Can you work these out from the model? Positions are in its coordinate system, mm. A direction names the side the tool comes from. Give positions to 0.01 mm unless a question says otherwise; leave off trailing zeros. Write each loop counter-clockwise with the first axis right and the second up, starting at its lowest first coordinate (ties: lowest second). Pieces come first, ordered by that corner, then holes.
1. Suppose I cut it at B-B (x = 1.75). Please give me the cut outline in (y, z), and give its area (3 significant figures).
2. Thinking about a two-plate mould opening in Z: for faces 3 (the flat face through (2, -4, 115.167)), 4 (the flat face through (2, -43.98, 30)), 5 (the cylindrical face through (1.6, 5.9, 103.3)), 6 (the cylindrical face through (1.6, 5.9, 27.1)), which applies, pulls with the +Z half, pulls with the -Z half, needs draft (parallel to the pull), parting line crosses it, or undercut?
3. I'm going to push a flat-ended pin straight in: pin 1 (3 mm diameter, centred on y = -31.21, z = 54.84, fed in from +X). Where does the tip first touch, or does it pass through?
4. Suppose I cut it at A-A (z = -11). Please give me the cut outline in (x, y) (3 decimals), and give its area (3 significant figures).
5. On a 3-axis mill with a long thin cutter (end or side, diameter ignored), from which of +Z, -Z, +X, -X, +Y, -Y can I reach the whole of each face in a straight line? I mean faces 1 (the flat face through (2, 44.989, 31)), 2 (the flat face through (2, -24.93, 30)). Say none if no direction works.
6. If I drill on probe 1 along Y at (x, z) = (1.15, -33); probe 2 along Z at (x, y) = (3.05, 8); probe 3 along Z at (x, y) = (2, 41.5), over which ranges is the centre line in solid material (lowest first)?
```python
from build123d import *

# Parameters (mm, degrees)
SKETCH1_R           = 2.54
BOSS_EXTRUDE1_DEPTH = 3.175


with BuildPart() as part:
    # Sketch1 → Boss-Extrude1 (new body)
    with BuildSketch(Plane(origin=(0, 0, 0), x_dir=(0, 0, -1), z_dir=(1, 0, 0))):
        Polygon((53.108364313, 44.988743573), (-118.341635687, 44.988743573), (-118.341635687, -56.611256427), (53.108364313, -56.611256427), (53.108364313, -55.023756427), (-115.166635687, -55.023756427), (-115.166635687, -53.504836427), (53.108364313, -53.504836427), (53.108364313, -50.261256427), (53.108364313, -43.979836427), (-115.166635687, -43.979836427), (-115.166635687, -37.629836427), (53.108364313, -37.629836427), (53.108364313, -24.929836427), (-115.166635687, -24.929836427), (-115.166635687, -18.579836427), (53.108364313, -18.579836427), (53.108364313, -5.879836427), (-115.166635687, -5.879836427), (-115.166635687, -2.704836427), (53.108364313, -2.704836427), (53.108364313, 25.938743573), (53.108364313, 40.226243573), (-115.166635687, 40.226243573), (-115.166635687, 43.401243573), (53.108364313, 43.401243573), align=None)
        with Locations((-54.841635687, -31.211256427)):
            Circle(SKETCH1_R, mode=Mode.SUBTRACT)
        with Locations((-105.641635687, 6.888743573)):
            Circle(SKETCH1_R, mode=Mode.SUBTRACT)
        with Locations((-29.441635687, 6.888743573)):
            Circle(SKETCH1_R, mode=Mode.SUBTRACT)
    extrude(amount=BOSS_EXTRUDE1_DEPTH)


solid = part.part
```
Checks:
1. outline: (-56.61, -53.11) - (-55.02, -53.11) - (-55.02, 115.17) - (-53.5, 115.17) - (-53.5, -53.11) - (-43.98, -53.11) - (-43.98, 115.17) - (-37.63, 115.17) - (-37.63, -53.11) - (-24.93, -53.11) - (-24.93, 115.17) - (-18.58, 115.17) - (-18.58, -53.11) - (-5.88, -53.11) - (-5.88, 115.17) - (-2.7, 115.17) - (-2.7, -53.11) - (40.23, -53.11) - (40.23, 115.17) - (43.4, 115.17) - (43.4, -53.11) - (44.99, -53.11) - (44.99, 118.34) - (-56.61, 118.34) - close; hole circle Ø5.08 at (-31.21, 54.84); hole circle Ø5.08 at (6.89, 29.44); hole circle Ø5.08 at (6.89, 105.64)
1. area: 13,900 mm2
2. face 3: pulls with the -Z half
2. face 4: needs draft
2. face 5: undercut
2. face 6: undercut
3. pin 1: passes through
4. outline: (0, -56.611) - (3.175, -56.611) - (3.175, -55.024) - (0, -55.024) - close; (0, -53.505) - (3.175, -53.505) - (3.175, -43.98) - (0, -43.98) - close; (0, -37.63) - (3.175, -37.63) - (3.175, -24.93) - (0, -24.93) - close; (0, -18.58) - (3.175, -18.58) - (3.175, -5.88) - (0, -5.88) - close; (0, -2.705) - (3.175, -2.705) - (3.175, 40.226) - (0, 40.226) - close; (0, 43.401) - (3.175, 43.401) - (3.175, 44.989) - (0, 44.989) - close
4. area: 257 mm2
5. face 1: +Z, -Z, +X, -X, +Y
5. face 2: -Z, +X, -X
6. probe 1: y = -56.61 to -55.02, -53.5 to -43.98, -37.63 to -24.93, -18.58 to -5.88, -2.7 to 40.23, 43.4 to 44.99
6. probe 2: z = -53.11 to 27.16, 31.73 to 103.36, 107.93 to 118.34
6. probe 3: z = 115.17 to 118.34
